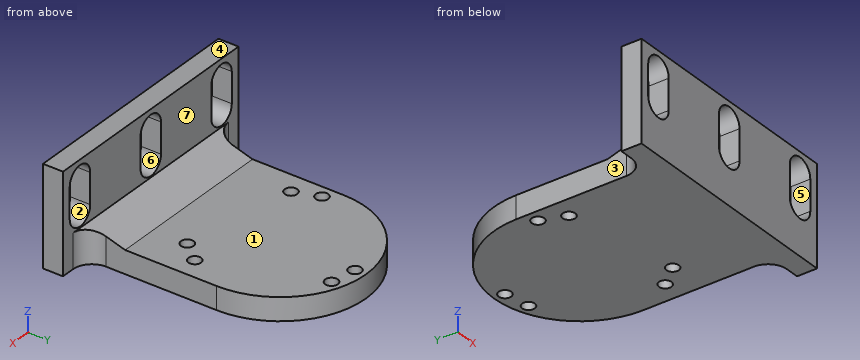
from build123d import *

# Parameters (mm, degrees)
SKETCH_1_R          = 1.65
EXTRUDE_1_DEPTH     = 6
SKETCH_2_W          = 62
SKETCH_2_H          = 5.25
EXTRUDE_2_DEPTH     = 26
CUT_EXTRUDE_1_DEPTH = 70.492805383
EXTRUDE_3_DEPTH     = 22.5
FILLET_1_R          = 5


with BuildPart() as part:
    # 스케치1 → 보스-돌출1 (new body)
    with BuildSketch(Plane.XY):
        with BuildLine():
            ThreePointArc((-22.5, 0), (0, 22.5), (22.5, 0))
            Line((22.5, 0), (22.5, -34))
            Line((22.5, -34), (-22.5, -34))
            Line((-22.5, -34), (-22.5, 0))
        make_face()
        with Locations((-19.32389773, -3.407324542)):
            Circle(SKETCH_1_R, mode=Mode.SUBTRACT)
        with Locations((16.993150473, -9.811)):
            Circle(SKETCH_1_R, mode=Mode.SUBTRACT)
        with Locations((6.711119252, 18.438648605)):
            Circle(SKETCH_1_R, mode=Mode.SUBTRACT)
        with Locations((0, 19.622)):
            Circle(SKETCH_1_R, mode=Mode.SUBTRACT)
        with Locations((12.612778477, -15.031324063)):
            Circle(SKETCH_1_R, mode=Mode.SUBTRACT)
        with Locations((-16.993150473, -9.811)):
            Circle(SKETCH_1_R, mode=Mode.SUBTRACT)
    extrude(amount=EXTRUDE_1_DEPTH)

    # 스케치2 → 보스-돌출2 (add)
    with BuildSketch(Plane.XY):
        with Locations((0, -36.625)):
            Rectangle(SKETCH_2_W, SKETCH_2_H)
    extrude(amount=EXTRUDE_2_DEPTH)

    # 스케치3 → 컷-돌출1 (cut, through all)
    with BuildSketch(Plane(origin=(0, -34, 0), x_dir=(1, 0, 0), z_dir=(0, 1, 0))):
        with BuildLine():
            Line((-3.625, -21), (-3.625, -13))
            ThreePointArc((-3.625, -13), (0, -9.375), (3.625, -13))
            Line((3.625, -13), (3.625, -21))
            ThreePointArc((3.625, -21), (0, -24.625), (-3.625, -21))
        make_face()
        with BuildLine():
            Line((21.375, -21), (21.375, -13))
            ThreePointArc((21.375, -13), (25, -9.375), (28.625, -13))
            Line((28.625, -13), (28.625, -21))
            ThreePointArc((28.625, -21), (25, -24.625), (21.375, -21))
        make_face()
        with BuildLine():
            Line((-28.625, -21), (-28.625, -13))
            ThreePointArc((-28.625, -13), (-25, -9.375), (-21.375, -13))
            Line((-21.375, -13), (-21.375, -21))
            ThreePointArc((-21.375, -21), (-25, -24.625), (-28.625, -21))
        make_face()
    extrude(amount=-CUT_EXTRUDE_1_DEPTH, mode=Mode.SUBTRACT)

    # 스케치4 → 보스-돌출3 (add, symmetric)
    with BuildSketch(Plane(origin=(0, 0, 0), x_dir=(0, 0, -1), z_dir=(1, 0, 0))):
        Polygon((-6, -24), (-9, -34), (-6, -34), align=None)
    extrude(amount=EXTRUDE_3_DEPTH, both=True)

    # 필렛1
    fillet_1_edges = [part.edges().sort_by_distance(p)[0] for p in [
        (22.5, -34, 4.5),
        (-22.5, -34, 4.5),
    ]]
    fillet(fillet_1_edges, radius=FILLET_1_R)


solid = part.part
Check sheet for the modelled part. Datum: model origin and axes. Units: mm. Face numbers are marked on the shaded views. A direction names the side the tool comes from. Give positions to 0.01 mm unless a question says otherwise; leave off trailing zeros. Loops run counter-clockwise (first coordinate to the right, second up) from the corner with the lowest first, then second, coordinate; pieces in that order, holes last. Notation, with made-up numbers: M -32,36 L 24,36 A12 cw 24,47 Z; hole C 51.5,9 d3. An arc over 180 degrees is marked long. Answer as a JSON object with one key per item and string values. Group by question number.
Q1. Material ranges on line 1 along X through (y, z) = (-35.5, 17.25) (3 decimals); line 2 along Y through (x, z) = (0, 1.5); line 3 along Z through (x, y) = (-11.5, -23), recorded low to high. Write a range as [from, to].
Q2. Release check for a two-part mould opening along Z. For the marked faces 4, 5, 6 and 7 record: released by +Z, released by -Z, zero draft, split by the parting line, or undercut.
Q3. Cross-section at D-D on x = 25. Record the cut outline in (y, z) (3 decimals), then the cut area to 3 significant figures.
Q4. Cross-section at B-B on z = 19.5. Record the cut outline in (x, y) (3 decimals).
Q5. Cross-section at A-A on x = 0. Record the cut outline in (y, z) (3 decimals).
Q6. Cross-section at C-C on y = -2.5. Record the cut outline in (x, z).
Q7. Go/stop test with flat-tipped pins: P1, Ø4, axis at y = -12.5, z = 2.5, coming from the -X side; P2, Ø22.5, axis at x = 0.5, y = -8, coming from the +Z side; P3, Ø13, axis at x = -1.5, z = 8, coming from the +Y side. Record where each tip stops, or that it passes through.
Q8. Access from +Z, -Z, +X, -X, +Y, -Y to the whole of each face (thin tool, end or side, straight path). Record for the marked faces 1, 2 and 3.
Evaluation:
{
 "1": {"line 1": "x = [-31, -28.625], [-21.375, -3.625], [3.625, 21.375], [28.625, 31]", "line 2": "y = [-39.25, 17.97], [21.27, 22.5]", "line 3": "z = [0, 6]"},
 "2": {"face 4": "released by +Z", "face 5": "undercut", "face 6": "undercut", "face 7": "zero draft"},
 "3": {"outline": "M -39.25,0 L -33.33,0 L -33.33,8.799 L -34,9 L -34,9.375 L -39.25,9.375 Z; M -39.25,24.625 L -34,24.625 L -34,26 L -39.25,26 Z", "area": "62.4 mm2"},
 "4": {"outline": "M -31,-39.25 L -28.625,-39.25 L -28.625,-34 L -31,-34 Z; M -21.375,-39.25 L -3.625,-39.25 L -3.625,-34 L -21.375,-34 Z; M 3.625,-39.25 L 21.375,-39.25 L 21.375,-34 L 3.625,-34 Z; M 28.625,-39.25 L 31,-39.25 L 31,-34 L 28.625,-34 Z"},
 "5": {"outline": "M -39.25,0 L 17.972,0 L 17.972,6 L -24,6 L -34,9 L -34,9.375 L -39.25,9.375 Z; M -39.25,24.625 L -34,24.625 L -34,26 L -39.25,26 Z; M 21.272,0 L 22.5,0 L 22.5,6 L 21.272,6 Z"},
 "6": {"outline": "M -22.5,0 L -20.7,0 L -20.7,6 L -22.5,6 Z; M -17.95,0 L 22.5,0 L 22.5,6 L -17.95,6 Z"},
 "7": {"P1": "stops at x = -22.5", "P2": "stops at z = 6", "P3": "stops at y = 22.5"},
 "8": {"face 1": "+Z, +X, -X, +Y", "face 2": "+Y, -Y", "face 3": "+Z, -Z, -X, +Y"}
}
